Build history of the part. All positions in model axes, mm. Give positions to 0.01 mm unless a question says otherwise; leave off trailing zeros. Loops run counter-clockwise (first coordinate to the right, second up) from the corner with the lowest first, then second, coordinate; pieces in that order, holes last.
1) Band-saw the part on A-A on y = 11. List the corners of the cut face in (x, z), then the cut area to 3 significant figures.
2) Flat gauge pins, fed straight in: P1, Ø6, axis at x = 1402.5, z = 12982, coming from the -Y side (3 decimals); P2, Ø4, axis at y = 3, z = 13010, coming from the +X side; P3, Ø4, axis at x = 1368, z = 13038, coming from the -Y side; P4, Ø3, axis at x = 1264.5, y = 5, coming from the -Z side. Where does each tip first touch, or does it go through?
3) Band-saw the part on B-B on z = 12895.5. List the corners of the cut face in (x, y).
4) Band-saw the part on C-C on x = 1188. List the corners of the cut face in (y, z).
5) Wall check: line 1 (X direction, y = 8.75, z = 13057); line 2 (X direction, y = 11, z = 12986); line 3 (Z direction, x = 1220.5, y = 15.5). Give the ranges that are in metal, low to high.
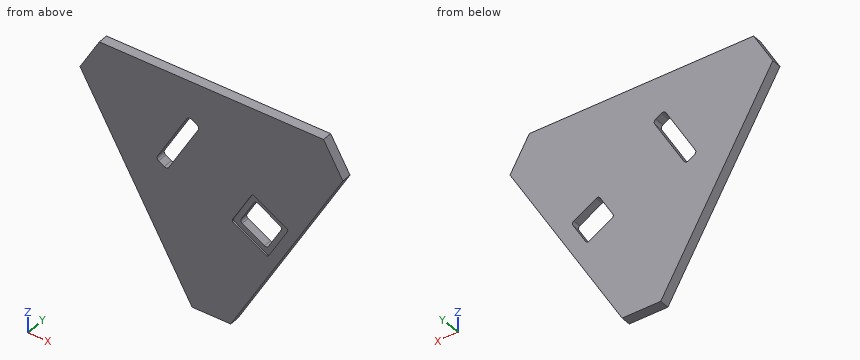
```python
from build123d import *

# Parameters (mm, degrees)
BOSS_EXTRUDE1_DEPTH = 19.05
CUT_EXTRUDE1_DEPTH  = 20
CUT_EXTRUDE2_DEPTH  = 3.175
CUT_EXTRUDE3_DEPTH  = 19.05


with BuildPart() as part:
    # Sketch1 → Boss-Extrude1 (new body)
    with BuildSketch(Plane(origin=(-388.281715987, 0, -288.185661777), x_dir=(1, 0, 0), z_dir=(0, 1, 0))):
        Polygon((1747.570833697, -13084.824581071), (1672.514355591, -13084.824581071), (1454.703489965, -13462.084066777), (1492.231729019, -13527.084883536), (1927.853460271, -13527.084883536), (1965.381699324, -13462.084066777), align=None)
    extrude(amount=BOSS_EXTRUDE1_DEPTH)

    # Sketch4 → Cut-Extrude1 (cut)
    with BuildSketch(Plane(origin=(0, 19.05, 0), x_dir=(1, 0, 0), z_dir=(0, 1, 0))):
        with BuildLine():
            Line((1377.232664741, -13008.917958926), (1402.232664763, -13052.21922919))
            ThreePointArc((1402.232664763, -13052.21922919), (1405.572299736, -13054.781821235), (1409.745804474, -13054.232368895))
            Line((1409.745804474, -13054.232368895), (1453.047074654, -13029.232368878))
            ThreePointArc((1453.047074654, -13029.232368878), (1455.609666681, -13025.892733929), (1455.060214377, -13021.7192292))
            Line((1455.060214377, -13021.7192292), (1430.060214339, -12978.417958945))
            ThreePointArc((1430.060214339, -12978.417958945), (1426.720579378, -12975.855366909), (1422.547074644, -12976.404819231))
            Line((1422.547074644, -12976.404819231), (1379.245804465, -13001.404819247))
            ThreePointArc((1379.245804465, -13001.404819247), (1376.683212438, -13004.744454197), (1377.232664741, -13008.917958926))
        make_face()
    extrude(amount=-CUT_EXTRUDE1_DEPTH, mode=Mode.SUBTRACT)

    # Sketch5 → Cut-Extrude2 (cut)
    with BuildSketch(Plane.XZ):
        with BuildLine():
            Line((1427.670911631, 12961.899565184), (1364.121967469, 12998.589565203))
            ThreePointArc((1364.121967469, 12998.589565203), (1362.34679007, 13000.903021429), (1362.72741068, 13003.794121991))
            Line((1362.72741068, 13003.794121991), (1399.417410699, 13067.343066154))
            ThreePointArc((1399.417410699, 13067.343066154), (1401.730866926, 13069.118243552), (1404.621967488, 13068.737622942))
            Line((1404.621967488, 13068.737622942), (1468.17091165, 13032.047622923))
            ThreePointArc((1468.17091165, 13032.047622923), (1469.946089048, 13029.734166696), (1469.565468439, 13026.843066135))
            Line((1469.565468439, 13026.843066135), (1432.87546842, 12963.294121972))
            ThreePointArc((1432.87546842, 12963.294121972), (1430.562012193, 12961.518944574), (1427.670911631, 12961.899565184))
        make_face()
    extrude(amount=-CUT_EXTRUDE2_DEPTH, mode=Mode.SUBTRACT)

    # Sketch6 → Cut-Extrude3 (cut)
    with BuildSketch(Plane(origin=(0, 19.05, 0), x_dir=(1, 0, 0), z_dir=(0, 1, 0))):
        with BuildLine():
            Line((1216.964435014, -13064.325242236), (1274.114435014, -13163.311945889))
            ThreePointArc((1274.114435014, -13163.311945889), (1277.970195391, -13166.270574886), (1282.788696328, -13165.636207203))
            Line((1282.788696328, -13165.636207203), (1293.787218956, -13159.286207203))
            ThreePointArc((1293.787218956, -13159.286207203), (1296.745847953, -13155.430446825), (1296.11148027, -13150.611945889))
            Line((1296.11148027, -13150.611945889), (1238.96148027, -13051.625242236))
            ThreePointArc((1238.96148027, -13051.625242236), (1235.105719892, -13048.66661324), (1230.287218956, -13049.300980922))
            Line((1230.287218956, -13049.300980922), (1219.288696328, -13055.650980922))
            ThreePointArc((1219.288696328, -13055.650980922), (1216.330067331, -13059.5067413), (1216.964435014, -13064.325242236))
        make_face()
    extrude(amount=-CUT_EXTRUDE3_DEPTH, mode=Mode.SUBTRACT)


solid = part.part
```
Findings below:
1. outline: (1066.42, 13173.9) - (1284.23, 12796.64) - (1359.29, 12796.64) - (1577.1, 13173.9) - (1539.57, 13238.9) - (1103.95, 13238.9) - close; hole (1216.96, 13064.33) arc R6.35 ccw to (1219.29, 13055.65) - (1230.29, 13049.3) arc R6.35 ccw to (1238.96, 13051.63) - (1296.11, 13150.61) arc R6.35 ccw to (1293.79, 13159.29) - (1282.79, 13165.64) arc R6.35 ccw to (1274.11, 13163.31) - close; hole (1377.23, 13008.92) arc R5.5 ccw to (1379.25, 13001.4) - (1422.55, 12976.4) arc R5.5 ccw to (1430.06, 12978.42) - (1455.06, 13021.72) arc R5.5 ccw to (1453.05, 13029.23) - (1409.75, 13054.23) arc R5.5 ccw to (1402.23, 13052.22) - close
1. area: 134,000 mm2
2. P1: stops at y = 3.175
2. P2: stops at x = 1483.63
2. P3: stops at y = 0
2. P4: stops at z = 12828.22
3. outline: (1227.16, 0) - (1416.37, 0) - (1416.37, 19.05) - (1227.16, 19.05) - close
4. outline: (0, 12963.32) - (19.05, 12963.32) - (19.05, 13238.9) - (0, 13238.9) - close
5. line 1: x = 1133.91 to 1217.66, 1242.06 to 1509.61
5. line 2: x = 1174.9 to 1405.93, 1434.44 to 1468.62
5. line 3: z = 12907.03 to 13054.95, 13070.45 to 13238.9
